from build123d import *

# Parameters (mm, degrees)
SKETCH1_R                        = 209.55
BOSS_EXTRUDE1_DEPTH              = 12.7
F_3_8_16_TAPPED_HOLE1_D          = 7.9375
F_3_8_16_TAPPED_HOLE1_DEPTH      = 19.304
F_3_8_16_TAPPED_HOLE1_TIP        = 2.384665582
CUT_EXTRUDE1_REACH               = 27.4
SKETCH4_R                        = 19.05
CUT_EXTRUDE2_REACH               = 27.4
SKETCH5_R                        = 12.7
CUT_EXTRUDE3_REACH               = 27.4
SKETCH6_R                        = 19.05
F_1_4_20_TAPPED_HOLE1_AT_2_COUNT = 2
F_1_4_20_TAPPED_HOLE1_AT_2_PITCH = 50.8
F_1_4_20_TAPPED_HOLE2_AT_2_COUNT = 2
F_1_4_20_TAPPED_HOLE2_AT_2_PITCH = 88.9
F_1_4_20_TAPPED_HOLE3_AT_2_COUNT = 2
F_1_4_20_TAPPED_HOLE3_AT_2_PITCH = 50.8
F_1_4_20_TAPPED_HOLE3_AT_3_COUNT = 2
F_1_4_20_TAPPED_HOLE3_AT_3_PITCH = 71.842048969
F_1_4_20_TAPPED_HOLE3_AT_4_COUNT = 2
F_1_4_20_TAPPED_HOLE3_AT_4_PITCH = 50.8


with BuildPart() as part:
    # Sketch1 → Boss-Extrude1 (new body, symmetric)
    with BuildSketch(Plane(origin=(0, 0, 0), x_dir=(1, 0, 0), z_dir=(0, 1, 0))):
        Circle(SKETCH1_R)
    extrude(amount=BOSS_EXTRUDE1_DEPTH, both=True)

    # 3/8-16 Tapped Hole1
    with Locations(Plane(origin=(0, -12.7, 0), x_dir=(-1, 0, 0), z_dir=(0, -1, 0))):
        with Locations((88.9, -88.9), (-88.9, -88.9), (-88.9, 88.9), (88.9, 88.9)):
            Hole(F_3_8_16_TAPPED_HOLE1_D / 2, depth=F_3_8_16_TAPPED_HOLE1_DEPTH)
            with Locations((0, 0, -(F_3_8_16_TAPPED_HOLE1_DEPTH + F_3_8_16_TAPPED_HOLE1_TIP / 2))):  # 118° drill point
                Cone(0, F_3_8_16_TAPPED_HOLE1_D / 2, F_3_8_16_TAPPED_HOLE1_TIP, mode=Mode.SUBTRACT)

    # Sketch4 → Cut-Extrude1 (cut, up to next)
    with BuildSketch(Plane(origin=(0, 12.7, 0), x_dir=(1, 0, 0), z_dir=(0, 1, 0)), mode=Mode.PRIVATE) as cut_extrude1_sk1:
        Circle(SKETCH4_R)
    cut_extrude1_tool1 = extrude(cut_extrude1_sk1.sketch, amount=-CUT_EXTRUDE1_REACH, mode=Mode.PRIVATE) & part.part
    add(cut_extrude1_tool1.solids().sort_by_distance((0, 12.7, 0))[0], mode=Mode.SUBTRACT)

    # Sketch5 → Cut-Extrude2 (cut, up to next)
    with BuildSketch(Plane(origin=(0, 12.7, 0), x_dir=(1, 0, 0), z_dir=(0, 1, 0)), mode=Mode.PRIVATE) as cut_extrude2_sk1:
        with Locations((0, -133.35)):
            Circle(SKETCH5_R)
    cut_extrude2_tool1 = extrude(cut_extrude2_sk1.sketch, amount=-CUT_EXTRUDE2_REACH, mode=Mode.PRIVATE) & part.part
    add(cut_extrude2_tool1.solids().sort_by_distance((0, 12.7, 133.35))[0], mode=Mode.SUBTRACT)
    # Sketch5 → Cut-Extrude2 (cut, up to next)
    with BuildSketch(Plane(origin=(0, 12.7, 0), x_dir=(1, 0, 0), z_dir=(0, 1, 0)), mode=Mode.PRIVATE) as cut_extrude2_sk2:
        with Locations((82.55, 133.35)):
            Circle(SKETCH5_R)
    cut_extrude2_tool2 = extrude(cut_extrude2_sk2.sketch, amount=-CUT_EXTRUDE2_REACH, mode=Mode.PRIVATE) & part.part
    add(cut_extrude2_tool2.solids().sort_by_distance((82.55, 12.7, -133.35))[0], mode=Mode.SUBTRACT)

    # Sketch6 → Cut-Extrude3 (cut, up to next)
    with BuildSketch(Plane(origin=(0, 12.7, 0), x_dir=(1, 0, 0), z_dir=(0, 1, 0)), mode=Mode.PRIVATE) as cut_extrude3_sk1:
        with Locations((-82.55, 133.35)):
            Circle(SKETCH6_R)
    cut_extrude3_tool1 = extrude(cut_extrude3_sk1.sketch, amount=-CUT_EXTRUDE3_REACH, mode=Mode.PRIVATE) & part.part
    add(cut_extrude3_tool1.solids().sort_by_distance((-82.55, 12.7, -133.35))[0], mode=Mode.SUBTRACT)

    # Sketch7 → 1/4-20 Tapped Hole1 (revolve, cut)
    with BuildSketch(Plane(origin=(-111.125, 12.7, -36.83), x_dir=(0, 0, 1), z_dir=(1, 0, 0))):
        Polygon((0, 0), (0, 20.583816902), (2.5527, 19.05), (2.5527, 0), align=None)
    f_1_4_20_tapped_hole1 = revolve(axis=Axis((-111.125, 19.05, -36.83), (0, -1, 0)), mode=Mode.SUBTRACT)

    # 1/4-20 Tapped Hole1 at 2: 1/4-20 Tapped Hole1 ×2
    with Locations(*[(i * F_1_4_20_TAPPED_HOLE1_AT_2_PITCH, 0, 0) for i in range(1, F_1_4_20_TAPPED_HOLE1_AT_2_COUNT)]):
        add(f_1_4_20_tapped_hole1, mode=Mode.SUBTRACT)

    # Sketch9 → 1/4-20 Tapped Hole2 (revolve, cut)
    with BuildSketch(Plane(origin=(-38.1, 12.7, -88.9), x_dir=(0, 0, 1), z_dir=(1, 0, 0))):
        Polygon((0, 0), (0, 20.583816902), (2.5527, 19.05), (2.5527, 0), align=None)
    f_1_4_20_tapped_hole2 = revolve(axis=Axis((-38.1, 19.05, -88.9), (0, -1, 0)), mode=Mode.SUBTRACT)

    # 1/4-20 Tapped Hole2 at 2: 1/4-20 Tapped Hole2 ×2
    with Locations(*[(-i * F_1_4_20_TAPPED_HOLE2_AT_2_PITCH, 0, 0) for i in range(1, F_1_4_20_TAPPED_HOLE2_AT_2_COUNT)]):
        add(f_1_4_20_tapped_hole2, mode=Mode.SUBTRACT)

    # Mirror1: 1/4-20 Tapped Hole2, 1/4-20 Tapped Hole1 across plane
    add(f_1_4_20_tapped_hole2.mirror(Plane(origin=(0, 0, 0), x_dir=(0, 0, 1), z_dir=(1, 0, 0))), mode=Mode.SUBTRACT)
    add(f_1_4_20_tapped_hole1.mirror(Plane(origin=(0, 0, 0), x_dir=(0, 0, 1), z_dir=(1, 0, 0))), mode=Mode.SUBTRACT)

    # Mirror1 copy 1 sketch → Mirror1 copy 1 (revolve, cut)
    with BuildSketch(Plane(origin=(127, 12.7, -88.9), x_dir=(0, 0, 1), z_dir=(-1, 0, 0))):
        Polygon((0, 0), (0, -20.583816902), (2.5527, -19.05), (2.5527, 0), align=None)
    revolve(axis=Axis((127, 19.05, -88.9), (0, 1, 0)), mode=Mode.SUBTRACT)

    # Mirror1 copy 2 sketch → Mirror1 copy 2 (revolve, cut)
    with BuildSketch(Plane(origin=(60.325, 12.7, -36.83), x_dir=(0, 0, 1), z_dir=(-1, 0, 0))):
        Polygon((0, 0), (0, -20.583816902), (2.5527, -19.05), (2.5527, 0), align=None)
    revolve(axis=Axis((60.325, 19.05, -36.83), (0, 1, 0)), mode=Mode.SUBTRACT)

    # Mirror2: 1/4-20 Tapped Hole2, 1/4-20 Tapped Hole1 across plane
    add(f_1_4_20_tapped_hole2.mirror(Plane.XY), mode=Mode.SUBTRACT)
    add(f_1_4_20_tapped_hole1.mirror(Plane.XY), mode=Mode.SUBTRACT)

    # Mirror2 copy 1 sketch → Mirror2 copy 1 (revolve, cut)
    with BuildSketch(Plane(origin=(38.1, 12.7, 88.9), x_dir=(0, 0, -1), z_dir=(-1, 0, 0))):
        Polygon((0, 0), (0, 20.583816902), (2.5527, 19.05), (2.5527, 0), align=None)
    revolve(axis=Axis((38.1, 19.05, 88.9), (0, -1, 0)), mode=Mode.SUBTRACT)

    # Mirror2 copy 2 sketch → Mirror2 copy 2 (revolve, cut)
    with BuildSketch(Plane(origin=(111.125, 12.7, 36.83), x_dir=(0, 0, -1), z_dir=(-1, 0, 0))):
        Polygon((0, 0), (0, 20.583816902), (2.5527, 19.05), (2.5527, 0), align=None)
    revolve(axis=Axis((111.125, 19.05, 36.83), (0, -1, 0)), mode=Mode.SUBTRACT)

    # Mirror2 copy 3 sketch → Mirror2 copy 3 (revolve, cut)
    with BuildSketch(Plane(origin=(127, 12.7, 88.9), x_dir=(0, 0, -1), z_dir=(-1, 0, 0))):
        Polygon((0, 0), (0, 20.583816902), (2.5527, 19.05), (2.5527, 0), align=None)
    revolve(axis=Axis((127, 19.05, 88.9), (0, -1, 0)), mode=Mode.SUBTRACT)

    # Mirror2 copy 4 sketch → Mirror2 copy 4 (revolve, cut)
    with BuildSketch(Plane(origin=(60.325, 12.7, 36.83), x_dir=(0, 0, -1), z_dir=(-1, 0, 0))):
        Polygon((0, 0), (0, 20.583816902), (2.5527, 19.05), (2.5527, 0), align=None)
    revolve(axis=Axis((60.325, 19.05, 36.83), (0, -1, 0)), mode=Mode.SUBTRACT)

    # Mirror2 copy 5 sketch → Mirror2 copy 5 (revolve, cut)
    with BuildSketch(Plane(origin=(-127, 12.7, 88.9), x_dir=(0, 0, -1), z_dir=(1, 0, 0))):
        Polygon((0, 0), (0, -20.583816902), (2.5527, -19.05), (2.5527, 0), align=None)
    revolve(axis=Axis((-127, 19.05, 88.9), (0, 1, 0)), mode=Mode.SUBTRACT)

    # Mirror2 copy 6 sketch → Mirror2 copy 6 (revolve, cut)
    with BuildSketch(Plane(origin=(-60.325, 12.7, 36.83), x_dir=(0, 0, -1), z_dir=(1, 0, 0))):
        Polygon((0, 0), (0, -20.583816902), (2.5527, -19.05), (2.5527, 0), align=None)
    revolve(axis=Axis((-60.325, 19.05, 36.83), (0, 1, 0)), mode=Mode.SUBTRACT)

    # Sketch12 → 1/4-20 Tapped Hole3 (revolve, cut)
    with BuildSketch(Plane(origin=(-177.8, -12.7, 25.4), x_dir=(0, 0, -1), z_dir=(1, 0, 0))):
        Polygon((0, 0), (0, 20.583816902), (2.5527, 19.05), (2.5527, 0), align=None)
    f_1_4_20_tapped_hole3 = revolve(axis=Axis((-177.8, -19.05, 25.4), (0, 1, 0)), mode=Mode.SUBTRACT)

    # 1/4-20 Tapped Hole3 at 2: 1/4-20 Tapped Hole3 ×2
    with Locations(*[(i * F_1_4_20_TAPPED_HOLE3_AT_2_PITCH, 0, 0) for i in range(1, F_1_4_20_TAPPED_HOLE3_AT_2_COUNT)]):
        add(f_1_4_20_tapped_hole3, mode=Mode.SUBTRACT)

    # 1/4-20 Tapped Hole3 at 3: 1/4-20 Tapped Hole3 ×2
    with Locations(*[Vector(0.707106781, 0, -0.707106781) * (i * F_1_4_20_TAPPED_HOLE3_AT_3_PITCH) for i in range(1, F_1_4_20_TAPPED_HOLE3_AT_3_COUNT)]):
        add(f_1_4_20_tapped_hole3, mode=Mode.SUBTRACT)

    # 1/4-20 Tapped Hole3 at 4: 1/4-20 Tapped Hole3 ×2
    with Locations(*[(0, 0, -i * F_1_4_20_TAPPED_HOLE3_AT_4_PITCH) for i in range(1, F_1_4_20_TAPPED_HOLE3_AT_4_COUNT)]):
        add(f_1_4_20_tapped_hole3, mode=Mode.SUBTRACT)

    # Mirror3: 1/4-20 Tapped Hole3 across plane
    add(f_1_4_20_tapped_hole3.mirror(Plane(origin=(0, 0, 0), x_dir=(0, 0, 1), z_dir=(1, 0, 0))), mode=Mode.SUBTRACT)

    # Mirror3 copy 1 sketch → Mirror3 copy 1 (revolve, cut)
    with BuildSketch(Plane(origin=(127, -12.7, 25.4), x_dir=(0, 0, -1), z_dir=(-1, 0, 0))):
        Polygon((0, 0), (0, -20.583816902), (2.5527, -19.05), (2.5527, 0), align=None)
    revolve(axis=Axis((127, -19.05, 25.4), (0, -1, 0)), mode=Mode.SUBTRACT)

    # Mirror3 copy 2 sketch → Mirror3 copy 2 (revolve, cut)
    with BuildSketch(Plane(origin=(127, -12.7, -25.4), x_dir=(0, 0, -1), z_dir=(-1, 0, 0))):
        Polygon((0, 0), (0, -20.583816902), (2.5527, -19.05), (2.5527, 0), align=None)
    revolve(axis=Axis((127, -19.05, -25.4), (0, -1, 0)), mode=Mode.SUBTRACT)

    # Mirror3 copy 3 sketch → Mirror3 copy 3 (revolve, cut)
    with BuildSketch(Plane(origin=(177.8, -12.7, -25.4), x_dir=(0, 0, -1), z_dir=(-1, 0, 0))):
        Polygon((0, 0), (0, -20.583816902), (2.5527, -19.05), (2.5527, 0), align=None)
    revolve(axis=Axis((177.8, -19.05, -25.4), (0, -1, 0)), mode=Mode.SUBTRACT)


solid = part.part
Could you check a few things on this model? Use its own coordinates, in mm. Give positions to 0.01 mm unless a question says otherwise; leave off trailing zeros. Order: outer loops, then holes, each group sorted by start corner. A loop starts at its lowest first (then second) coordinate and runs counter-clockwise, first axis right, second up.
1. For pin 1 (4 mm diameter, centred on y = -5.5, z = -55.5, fed in from -X); pin 2 (8 mm diameter, centred on x = -111.125, z = -36.83, fed in from +Y); pin 3 (5 mm diameter, centred on y = -1, z = 132.5, fed in from -X); pin 4 (4.5 mm diameter, centred on x = 127, z = 88.9, fed in from +Y), each with a flat end and sliding along its axis, tell me the tip position at first contact or that it passes through.
Answers below:
pin 1: stops at x = -202.61
pin 2: stops at y = 12.7
pin 3: stops at x = -164.35
pin 4: stops at y = -6.53
2. Suppose I cut it at C-C (z = 64). Write out the boundary of the cut face in (x, y), plus the area to 3 significant figures.
Answers below:
outline: (-199.54, -12.7) - (199.54, -12.7) - (199.54, 12.7) - (-199.54, 12.7) - close
area: 10,100 mm2
3. Suppose I cut it at B-B (x = 139). Write out the boundary of the cut face in (y, z), plus the area to 3 significant figures.
Answers below:
outline: (-12.7, -156.81) - (12.7, -156.81) - (12.7, 156.81) - (-12.7, 156.81) - close
area: 7,970 mm2
4. Suppose I cut it at A-A (y = 1.5). State how many separate pieces and enclosed holes the cut face has, plus the area to 3 significant figures.
Answers below:
separate pieces: 1
enclosed holes: 32
area: 134,000 mm2
5. I need wall thicknesses on L1, parallel to Z at x = 177.8, y = 1.5; L2, parallel to X at y = 0.5, z = 36.83; L3, parallel to Z at x = -88.5, y = 1. Which ranges of each line are inside material? Lowest first, please.
Answers below:
L1: z = -110.9 to -27.95, -22.85 to 22.85, 27.95 to 110.9
L2: x = -206.29 to -113.68, -108.57 to -62.88, -57.77 to 57.77, 62.88 to 108.57, 113.68 to 206.29
L3: z = -189.94 to -151.45, -115.25 to -92.85, -84.95 to 84.95, 92.85 to 189.94
6. Thinking about a two-plate mould opening in X: for faces 1 (the cylindrical face through (-15.12, 0.18, 11.59)), 2 (the flat face through (-3, 12.7, 44)), 3 (the cylindrical face through (-45.426, 0.178, 204.567)), 4 (the cylindrical face through (89.377, 0.178, -144.059)), which applies, +X half, -X half, draft (parallel to the pull), parting line (faces both ways), or undercut?
Answers below:
face 1: undercut
face 2: draft
face 3: parting line
face 4: undercut
